Build history of the part. All positions in model axes, mm. Face numbers are marked on the shaded views. A direction names the side the tool comes from. Give positions to 0.01 mm unless a question says otherwise; leave off trailing zeros. Order: outer loops, then holes, each group sorted by start corner. A loop starts at its lowest first (then second) coordinate and runs counter-clockwise, first axis right, second up. Notation, with made-up numbers: M -20.5,38 L 35.5,38 A21 ccw 35.5,60 Z; hole C 73.25,82 d8. An arc over 180 degrees is marked long. Use CSV: the item, a comma, the result in double quotes. Start each with the question number.
Item 1: Band-saw the part on B-B on z = 0.75. Give the number of separate pieces and of enclosed holes in the cut face, plus the area to 3 significant figures.
Item 2: Pin check, flat tips, straight feed: P1, Ø12, axis at x = -46.5, z = 4, coming from the +Y side; P2, Ø1.5, axis at x = -3.5, z = 3, coming from the -Y side; P3, Ø4, axis at y = 16, z = -4, coming from the -X side. Stop position of each tip, or through.
Item 3: Two-plate mould, pull along Y, no slides. Class the marked faces 5, 6, 7 and 8: pulls with the +Y half, pulls with the -Y half, needs draft (parallel to the pull), parting line crosses it, or undercut.
Item 4: Which spindle directions (+Z, -Z, +X, -X, +Y, -Y) get a long thin tool onto all of the face, cutting with end or side? Do the marked faces 1, 2, 3 and 4. Say none if no direction does.
Item 5: Band-saw the part on A-A on x = 91.5. Write the cut outline in (y, z), plus the area to 3 significant figures.
Item 6: Band-saw the part on C-C on y = -17. Write the cut outline in (x, z).
Item 7: Wall check: line 1 along X through (y, z) = (0.5, -1.5); line 2 along Y through (x, z) = (-75, -3.25); line 3 along Y through (x, z) = (11.5, 2.5). Give the ranges that are in metal, low to high.
Item 8: Band-saw the part on D-D on x = 25. Write the cut outline in (y, z), plus the area to 3 significant figures.
from build123d import *

# Parameters (mm, degrees)
CROQUIS1_W                            = 192
CROQUIS1_H                            = 20
SALIENTE_EXTRUIR1_DEPTH               = 10
TALADRO_DE_MARGEN_PARA_M81_D          = 10.2
TALADRO_DE_MARGEN_PARA_M81_DEPTH      = 200
TALADRO_DE_MARGEN_PARA_M81_TIP        = 3.064389157
CROQUIS5_W                            = 40
CROQUIS5_H                            = 2
CORTAR_EXTRUIR1_DEPTH                 = 20
TALADRO_DE_MARGEN_PARA_M51_AT_2_COUNT = 2
TALADRO_DE_MARGEN_PARA_M51_AT_2_PITCH = 17
CROQUIS10_R                           = 25
SALIENTE_EXTRUIR2_DEPTH               = 20
CROQUIS11_R                           = 10.25
CORTAR_EXTRUIR2_DEPTH                 = 30
REDONDEO1_R                           = 10
MATRIZC1_COUNT                        = 6


with BuildPart() as part:
    # Croquis1 → Saliente-Extruir1 (new, symmetric)
    with BuildSketch(Plane.XY):
        Rectangle(CROQUIS1_W, CROQUIS1_H)
    extrude(amount=SALIENTE_EXTRUIR1_DEPTH, both=True)

    # Taladro de margen para M81
    with Locations(Plane.XY.offset(10)):
        with Locations((-83, 0), (83, 0)):
            Hole(TALADRO_DE_MARGEN_PARA_M81_D / 2, depth=TALADRO_DE_MARGEN_PARA_M81_DEPTH)
            with Locations((0, 0, -(TALADRO_DE_MARGEN_PARA_M81_DEPTH + TALADRO_DE_MARGEN_PARA_M81_TIP / 2))):  # 118° drill point
                Cone(0, TALADRO_DE_MARGEN_PARA_M81_D / 2, TALADRO_DE_MARGEN_PARA_M81_TIP, mode=Mode.SUBTRACT)

    # Croquis5 → Cortar-Extruir1 (cut)
    with BuildSketch(Plane.XY.offset(10)):
        with Locations((-76, 0)):
            Rectangle(CROQUIS5_W, CROQUIS5_H)
    cortar_extruir1 = extrude(amount=-CORTAR_EXTRUIR1_DEPTH, mode=Mode.SUBTRACT)

    # Croquis8 → Taladro de margen para M51 (revolve, cut)
    with BuildSketch(Plane(origin=(-91.5, -10, 0), x_dir=(0, 0, -1), z_dir=(1, 0, 0))):
        Polygon((0, 0), (0, 201.59228064), (2.65, 200), (2.65, 0), align=None)
    taladro_de_margen_para_m51 = revolve(axis=Axis((-91.5, -16.35, 0), (0, 1, 0)), mode=Mode.SUBTRACT)

    # Taladro de margen para M51 at 2: Taladro de margen para M51 ×2
    with Locations(*[(i * TALADRO_DE_MARGEN_PARA_M51_AT_2_PITCH, 0, 0) for i in range(1, TALADRO_DE_MARGEN_PARA_M51_AT_2_COUNT)]):
        add(taladro_de_margen_para_m51, mode=Mode.SUBTRACT)

    # Simetría1: Cortar-Extruir1, Taladro de margen para M51 across plane
    add(cortar_extruir1.mirror(Plane(origin=(0, 0, 0), x_dir=(0, 0, 1), z_dir=(1, 0, 0))), mode=Mode.SUBTRACT)
    add(taladro_de_margen_para_m51.mirror(Plane(origin=(0, 0, 0), x_dir=(0, 0, 1), z_dir=(1, 0, 0))), mode=Mode.SUBTRACT)

    # Simetría1 copy 1 sketch → Simetría1 copy 1 (revolve, cut)
    with BuildSketch(Plane(origin=(74.5, -10, 0), x_dir=(0, 0, -1), z_dir=(-1, 0, 0))):
        Polygon((0, 0), (0, -201.59228064), (2.65, -200), (2.65, 0), align=None)
    revolve(axis=Axis((74.5, -16.35, 0), (0, -1, 0)), mode=Mode.SUBTRACT)

    # Croquis10 → Saliente-Extruir2 (add)
    with BuildSketch(Plane.XY.offset(10)):
        Circle(CROQUIS10_R)
    extrude(amount=-SALIENTE_EXTRUIR2_DEPTH)

    # Croquis11 → Cortar-Extruir2 (cut)
    with BuildSketch(Plane.XY.offset(10)):
        Circle(CROQUIS11_R)
    extrude(amount=-CORTAR_EXTRUIR2_DEPTH, mode=Mode.SUBTRACT)

    # Redondeo1
    redondeo1_edges = [part.edges().sort_by_distance(p)[0] for p in [
        (-22.912878475, 10, 0),
        (22.912878475, 10, 0),
        (-22.912878475, -10, 0),
        (22.912878475, -10, 0),
    ]]
    fillet(redondeo1_edges, radius=REDONDEO1_R)

    # Croquis12 → Taladro roscado M31 (revolve, cut)
    with BuildSketch(Plane(origin=(0, 14, 10), x_dir=(0, -1, 0), z_dir=(1, 0, 0))):
        Polygon((0, 0), (0, 20.751075774), (1.25, 20), (1.25, 0), align=None)
    taladro_roscado_m31 = revolve(axis=Axis((0, 14, 16.35), (0, 0, -1)), mode=Mode.SUBTRACT)

    # MatrizC1: Taladro roscado M31 ×6 about axis
    matrizc1_axis = Axis((0, 0, 0), (0, 0, 1))
    for i in range(1, MATRIZC1_COUNT):
        add(taladro_roscado_m31.rotate(matrizc1_axis, i * 360 / MATRIZC1_COUNT), mode=Mode.SUBTRACT)


solid = part.part
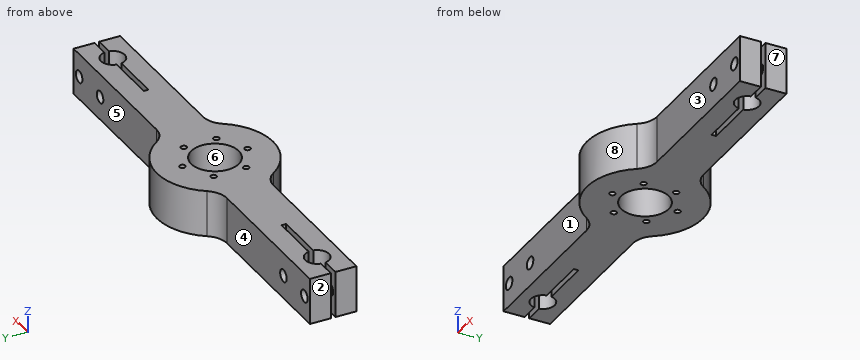
Model answer:
1,separate pieces,"9"
1,enclosed holes,"7"
1,area,"3,840 mm^2"
2,P1,"stops at y = 10"
2,P2,"stops at y = -24.85"
2,P3,"stops at x = -20.72"
3,face 5,"pulls with the +Y half"
3,face 6,"undercut"
3,face 7,"needs draft"
3,face 8,"pulls with the -Y half"
4,face 1,"+Z, -Z, -X, -Y"
4,face 2,"+Z, -Z, -X, +Y, -Y"
4,face 3,"+Z, -Z, +X, -Y"
4,face 4,"+Z, -Z, -X, +Y"
5,outline,"M -10,-10 L -1,-10 L -1,-2.65 L -10,-2.65 Z; M -10,2.65 L -1,2.65 L -1,10 L -10,10 Z; M 1,-10 L 10,-10 L 10,-2.65 L 1,-2.65 Z; M 1,2.65 L 10,2.65 L 10,10 L 1,10 Z"
5,area,"265 mm^2"
6,outline,"M -18.33,-10 L 18.33,-10 L 18.33,10 L -18.33,10 Z"
7,line 1,"x = -56 to -10.24, 10.24 to 56"
7,line 2,"y = -10 to -1, 1 to 10"
7,line 3,"y = -22.2 to -8.08, -5.92 to 5.92, 8.08 to 22.2"
8,outline,"M -10.72,-10 L 10.72,-10 L 10.72,10 L -10.72,10 Z"
8,area,"429 mm^2"
